```python
from build123d import *

# Parameters (mm, degrees)
SKETCH2_R           = 1.905
CUT_EXTRUDE1_DEPTH  = 4.318
CUT_EXTRUDE2_DEPTH  = 66.838691254
SKETCH4_R           = 4.699
BOSS_EXTRUDE1_DEPTH = 10.668


with BuildPart() as part:
    # Sketch1 → Revolve1 (revolve)
    with BuildSketch(Plane.XY, mode=Mode.PRIVATE) as revolve1_sk:
        Polygon((-42.799, 0), (0, 0), (0, 4.572), (-4.318, 4.572), (-4.318, 25.908), (-10.922, 25.908), (-10.922, 8.636), (-21.717, 8.636), (-21.717, 4.318), (-42.799, 4.318), align=None)
    revolve(revolve1_sk.sketch.rotate(Axis((0, 25.908, 0), (0, -1, 0)), 270), axis=Axis((0, 25.908, 0), (0, -1, 0)))

    # Sketch2 → Cut-Extrude1 (cut)
    with BuildSketch(Plane(origin=(0, 4.318, 0), x_dir=(1, 0, 0), z_dir=(0, 1, 0))):
        with Locations(Location((-31.001055742, 9.366043342, 0), (0, 0, 270))):
            Circle(SKETCH2_R)
        with Locations(Location((-22.164680145, 23.611759338, 0), (0, 0, 270))):
            Circle(SKETCH2_R)
        with Locations(Location((-7.389296403, 31.530723488, 0), (0, 0, 270))):
            Circle(SKETCH2_R)
        with Locations(Location((9.366043342, 31.001055742, 0), (0, 0, 270))):
            Circle(SKETCH2_R)
        with Locations(Location((23.611759338, 22.164680145, 0), (0, 0, 270))):
            Circle(SKETCH2_R)
        with Locations(Location((31.530723488, 7.389296403, 0), (0, 0, 270))):
            Circle(SKETCH2_R)
        with Locations(Location((31.001055742, -9.366043342, 0), (0, 0, 270))):
            Circle(SKETCH2_R)
        with Locations(Location((22.164680145, -23.611759338, 0), (0, 0, 270))):
            Circle(SKETCH2_R)
        with Locations(Location((7.389296403, -31.530723488, 0), (0, 0, 270))):
            Circle(SKETCH2_R)
        with Locations(Location((-9.366043342, -31.001055742, 0), (0, 0, 270))):
            Circle(SKETCH2_R)
        with Locations(Location((-23.611759338, -22.164680145, 0), (0, 0, 270))):
            Circle(SKETCH2_R)
        with Locations(Location((-31.530723488, -7.389296403, 0), (0, 0, 270))):
            Circle(SKETCH2_R)
    extrude(amount=-CUT_EXTRUDE1_DEPTH, mode=Mode.SUBTRACT)

    # Sketch3 → Cut-Extrude2 (cut, through all)
    with BuildSketch(Plane.XZ):
        with BuildLine():
            ThreePointArc((42.799, 0), (42.744006542, 2.168941149), (42.579167494, 4.33230845))
            Line((42.579167494, 4.33230845), (36.83, 0))
            Line((36.83, 0), (42.579167494, -4.33230845))
            ThreePointArc((42.579167494, -4.33230845), (42.744006542, -2.168941149), (42.799, 0))
        make_face()
        with BuildLine():
            Line((-36.83, 0), (-42.579167494, 4.33230845))
            ThreePointArc((-42.579167494, 4.33230845), (-42.799, 0), (-42.579167494, -4.33230845))
            Line((-42.579167494, -4.33230845), (-36.83, 0))
        make_face()
    extrude(amount=-CUT_EXTRUDE2_DEPTH, mode=Mode.SUBTRACT)

    # Sketch4 → Boss-Extrude1 (add)
    with BuildSketch(Plane.XZ):
        with Locations(Location((0, 32.385, 0), (0, 0, 90))):
            Circle(SKETCH4_R)
        with Locations(Location((32.385, 0, 0), (0, 0, 2.299654478))):
            Circle(SKETCH4_R)
        with Locations(Location((0, -32.385, 0), (0, 0, 90))):
            Circle(SKETCH4_R)
        with Locations(Location((-32.385, 0, 0), (0, 0, 177.700345522))):
            Circle(SKETCH4_R)
    extrude(amount=BOSS_EXTRUDE1_DEPTH)


solid = part.part
```
Model file for the job. Use its own axes, mm. A direction names the side the tool comes from. Give positions to 0.01 mm unless a question says otherwise; leave off trailing zeros. Order: outer loops, then holes, each group sorted by start corner. A loop starts at its lowest first (then second) coordinate and runs counter-clockwise, first axis right, second up.
1) Pin check, flat tips, straight feed: pin 1 (5 mm diameter, centred on x = 9.37, z = -31, fed in from -Y); pin 2 (3.5 mm diameter, centred on x = -22.16, z = -23.61, fed in from +Y); pin 3 (4 mm diameter, centred on x = 9, y = 3.5, fed in from +Z); pin 4 (5 mm diameter, centred on x = -7.39, z = -31.53, fed in from +Y). Stop position of each tip, or through.
2) Saw through at C-C, the plane z = -14.5. Write the cut outline in (x, y), then the cut area to 3 significant figures.
3) Saw through at D-D, the plane y = -4.5. Write the cut outline in (x, z) (3 decimals).
4) Saw through at A-A, the plane x = 0. Write the cut outline in (y, z).
5) Wall check: probe 1 along X at (y, z) = (1.5, 30); probe 2 along Y at (x, z) = (0.5, -11); probe 3 along Y at (x, z) = (-9, 36). Give the ranges that are in metal, low to high.
6) Saw through at B-B, the plane y = 14. Write the cut outline in (x, z), then the cut area to 3 significant figures.
7) 3-axis set-ups, long thin cutter, end or side, ignore diameter. For faces 1 (the flat face through (-10, 4.318, 20)), 2 (the cylindrical face through (-6.102, 2.189, -32.935)): which of +Z, -Z, +X, -X, +Y, -Y reach the whole face in a straight line?
8) Mould opens along Z. For faces 3 (the cylindrical face through (-36.92, -5.26, -1.23)), 4 (the flat face through (32, -10.668, 0)), 5 (the cylindrical face through (-29.92, 2.19, 8.41)) say: +Z half, -Z half, draft (parallel to the pull), parting line (faces both ways), or undercut.
Computed:
1. pin 1: stops at y = 0
1. pin 2: passes through
1. pin 3: stops at z = 42.22
1. pin 4: stops at y = 4.32
2. outline: (-40.27, 0) - (40.27, 0) - (40.27, 4.32) - (16.17, 4.32) - (16.17, 8.64) - (-16.17, 8.64) - (-16.17, 4.32) - (-40.27, 4.32) - close
2. area: 487 mm2
3. outline: circle Ø9.398 at (-32.385, 0); circle Ø9.398 at (0, -32.385); circle Ø9.398 at (0, 32.385); circle Ø9.398 at (32.385, 0)
4. outline: (-10.67, -37.08) - (0, -37.08) - (0, -42.8) - (4.32, -42.8) - (4.32, -21.72) - (8.64, -21.72) - (8.64, -10.92) - (25.91, -10.92) - (25.91, -4.32) - (4.57, -4.32) - (4.57, 4.32) - (25.91, 4.32) - (25.91, 10.92) - (8.64, 10.92) - (8.64, 21.72) - (4.32, 21.72) - (4.32, 42.8) - (0, 42.8) - (0, 37.08) - (-10.67, 37.08) - (-10.67, 27.69) - (0, 27.69) - (0, -27.69) - (-10.67, -27.69) - close
5. probe 1: x = -30.52 to -10.99, -7.75 to 6.26, 8.52 to 30.52
5. probe 2: y = 0 to 8.64
5. probe 3: y = 0 to 4.32
6. outline: circle Ø21.84 at (0, 0); hole circle Ø8.64 at (0, 0)
6. area: 316 mm2
7. face 1: +Y
7. face 2: +Y, -Y
8. face 3: parting line
8. face 4: draft
8. face 5: undercut
